from build123d import *

# Parameters (mm, degrees)
EXTRUDE_1_DEPTH              = 5
FILLET_1_R                   = 9
FILLET_2_R                   = 18
SHELL_1_T                    = -2
SKETCH_2_W                   = 27
SKETCH_2_H                   = 27
EXTRUDE_2_DEPTH              = 1
SKETCH_3_R                   = 3.975
EXTRUDE_3_DEPTH              = 1
FILLET_3_R                   = 3
HOLE_WIZARD_M2_1_D           = 2.1
HOLE_WIZARD_M2_1_CBORE_D     = 3.8
HOLE_WIZARD_M2_1_CBORE_DEPTH = 1
PATTERN_CIRCULAR_1_COUNT     = 4
SKETCH_6_R                   = 3.975
CUT_EXTRUDE_1_DEPTH          = 1
SKETCH_7_R                   = 2.5
CUT_EXTRUDE_2_DEPTH          = 2


with BuildPart() as part:
    # ｽｹｯﾁ1 → ﾎﾞｽ - 押し出し1 (new body)
    with BuildSketch(Plane(origin=(0, 0, 0), x_dir=(1, 0, 0), z_dir=(0, 1, 0))):
        with BuildLine():
            Line((-20, 50), (28.833147735, 50))
            ThreePointArc((28.833147735, 50), (44, 0), (28.833147735, -50))
            Line((28.833147735, -50), (-20, -50))
            Line((-20, -50), (-20, 50))
        make_face()
    extrude(amount=EXTRUDE_1_DEPTH)

    # ﾌｨﾚｯﾄ1
    fillet_1_edges = [part.edges().sort_by_distance(p)[0] for p in [
        (-20, 2.5, -50),
        (-20, 2.5, 50),
    ]]
    fillet(fillet_1_edges, radius=FILLET_1_R)

    # ﾌｨﾚｯﾄ2
    fillet_2_edges = [part.edges().sort_by_distance(p)[0] for p in [
        (28.833147735, 2.5, -50),
        (28.833147735, 2.5, 50),
    ]]
    fillet(fillet_2_edges, radius=FILLET_2_R)

    # ｼｪﾙ1
    shell_1_openings = [part.faces().sort_by_distance(p)[0] for p in [
        (9.782139289, 5, 0),
    ]]
    offset(amount=SHELL_1_T, openings=shell_1_openings, kind=Kind.INTERSECTION)

    # ｽｹｯﾁ2 → ﾎﾞｽ - 押し出し2 (add)
    with BuildSketch(Plane(origin=(0, 2, 0), x_dir=(1, 0, 0), z_dir=(0, 1, 0))):
        Rectangle(SKETCH_2_W, SKETCH_2_H)
    extrude(amount=EXTRUDE_2_DEPTH)

    # ｽｹｯﾁ3 → ﾎﾞｽ - 押し出し3 (add)
    with BuildSketch(Plane(origin=(0, 3, 0), x_dir=(1, 0, 0), z_dir=(0, 1, 0))):
        with Locations(Location((0, 0, 0), (0, 0, 270))):
            Circle(SKETCH_3_R)
    extrude(amount=EXTRUDE_3_DEPTH)

    # ﾌｨﾚｯﾄ3
    fillet_3_edges = [part.edges().sort_by_distance(p)[0] for p in [
        (13.5, 2.5, 13.5),
        (13.5, 2.5, -13.5),
        (-13.5, 2.5, -13.5),
        (-13.5, 2.5, 13.5),
    ]]
    fillet(fillet_3_edges, radius=FILLET_3_R)

    # M2 なべ頭ねじ用座ぐり穴1 (through all)
    with Locations(Plane(origin=(0, 0, 0), x_dir=(-1, 0, 0), z_dir=(0, -1, 0))):
        with Locations((10.5, 10.5)):
            hole_wizard_m2_1 = CounterBoreHole(HOLE_WIZARD_M2_1_D / 2, HOLE_WIZARD_M2_1_CBORE_D / 2, HOLE_WIZARD_M2_1_CBORE_DEPTH)

    # 円形ﾊﾟﾀｰﾝ1: M2 なべ頭ねじ用座ぐり穴1 ×4 about axis
    pattern_circular_1_axis = Axis((0, 0, 0), (0, 1, 0))
    for i in range(1, PATTERN_CIRCULAR_1_COUNT):
        add(hole_wizard_m2_1.rotate(pattern_circular_1_axis, i * 360 / PATTERN_CIRCULAR_1_COUNT), mode=Mode.SUBTRACT)

    # ｽｹｯﾁ6 → ｶｯﾄ - 押し出し1 (cut)
    with BuildSketch(Plane(origin=(0, 3, 0), x_dir=(1, 0, 0), z_dir=(0, 1, 0))):
        with BuildLine():
            Line((-7.994506037, -12.15), (7.994506037, -12.15))
            ThreePointArc((7.994506037, -12.15), (8.378679656, -8.378679656), (12.15, -7.994506037))
            Line((12.15, -7.994506037), (12.15, 7.994506037))
            ThreePointArc((12.15, 7.994506037), (8.378679656, 8.378679656), (7.994506037, 12.15))
            Line((7.994506037, 12.15), (-7.994506037, 12.15))
            ThreePointArc((-7.994506037, 12.15), (-7.62628447, 11.36125435), (-7.5, 10.5))
            ThreePointArc((-7.5, 10.5), (-9.076975053, 7.858977471), (-12.15, 7.994506037))
            Line((-12.15, 7.994506037), (-12.15, -7.994506037))
            ThreePointArc((-12.15, -7.994506037), (-9.076975053, -7.858977471), (-7.5, -10.5))
            ThreePointArc((-7.5, -10.5), (-7.62628447, -11.36125435), (-7.994506037, -12.15))
        make_face()
        with Locations(Location((0, 0, 0), (0, 0, 270))):
            Circle(SKETCH_6_R, mode=Mode.SUBTRACT)
    extrude(amount=-CUT_EXTRUDE_1_DEPTH, mode=Mode.SUBTRACT)

    # ｽｹｯﾁ7 → ｶｯﾄ - 押し出し2 (cut)
    with BuildSketch(Plane(origin=(0, 4, 0), x_dir=(1, 0, 0), z_dir=(0, 1, 0))):
        with Locations(Location((0, 0, 0), (0, 0, 270))):
            Circle(SKETCH_7_R)
    extrude(amount=-CUT_EXTRUDE_2_DEPTH, mode=Mode.SUBTRACT)


solid = part.part
Could you check a few things on this model? Use its own coordinates, in mm. A direction names the side the tool comes from. Coordinates: 2 decimals unless noted, no trailing zeros. Loops run counter-clockwise (first coordinate to the right, second up) from the corner with the lowest first, then second, coordinate; pieces in that order, holes last. Notation, with made-up numbers: (29.25, 45.25) -> (45.25, 45.25) arc R11 ccw to (45.25, 66.25) -> close; hole circle Ø4 at (74.5, 20). An arc over 180 degrees is marked (long way). Answer in a Markdown table with one row per item.
(1) Imagine slicing it at B-B (x = 19.5). List the corners of the cut face in (y, z) for me, plus the area to 3 significant figures.
Results found:
| item | result |
|---|---|
| outline | (0, -49.97) -> (5, -49.97) -> (5, -47.97) -> (2, -47.97) -> (2, 47.97) -> (5, 47.97) -> (5, 49.97) -> (0, 49.97) -> close |
| area | 212 mm^2 |
(2) If I drill on probe 1 along Z at (x, y) = (-10.5, 2.1); probe 2 along Z at (x, y) = (-10.5, 1.5); probe 3 along X at (y, z) = (1.6, -10.5), over which ranges is the centre line in solid material (lowest first)?
Results found:
| item | result |
|---|---|
| probe 1 | z = -50 to -48, -13.5 to -11.55, -9.45 to -7.5, 7.5 to 9.45, 11.55 to 13.5, 48 to 50 |
| probe 2 | z = -50 to -11.55, -9.45 to 9.45, 11.55 to 50 |
| probe 3 | x = -20 to -11.55, -9.45 to 9.45, 11.55 to 43.39 |
(3) Thinking about a two-plate mould opening in X: for faces 4 (the face through (12, 0, -1)), 5 (the face through (12, 1, 11)), 6 (the face through (-20, 2, 1)), which applies, released by +X, released by -X, zero draft, split by the parting line, or undercut?
Results found:
| item | result |
|---|---|
| face 4 | zero draft |
| face 5 | undercut |
| face 6 | released by -X |
(4) Will these pins go through, and if not, where does the flat tip stop? pin 1 Ø1.5 at (x, z) = (-3, -2.5) entering from +Y; pin 2 Ø1 at (x, y) = (22.5, 3) entering from -Z; pin 3 Ø2.5 at (x, z) = (-10.5, -10.5) entering from +Y; pin 4 Ø1.3 at (x, z) = (10.5, 10.5) entering from +Y.
Results found:
| item | result |
|---|---|
| pin 1 | stops at y = 4 |
| pin 2 | stops at z = -49.66 |
| pin 3 | stops at y = 3 |
| pin 4 | passes through |
(5) Imagine slicing it at A-A (z = 0). List the corners of the cut face in (x, y) for me (3 decimals).
Results found:
| item | result |
|---|---|
| outline | (-20, 0) -> (44, 0) -> (44, 5) -> (42, 5) -> (42, 2) -> (13.5, 2) -> (13.5, 3) -> (12.15, 3) -> (12.15, 2) -> (3.975, 2) -> (3.975, 4) -> (2.5, 4) -> (2.5, 2) -> (-2.5, 2) -> (-2.5, 4) -> (-3.975, 4) -> (-3.975, 2) -> (-12.15, 2) -> (-12.15, 3) -> (-13.5, 3) -> (-13.5, 2) -> (-18, 2) -> (-18, 5) -> (-20, 5) -> close |
(6) For faces 1 (the face through (28.103, 2.535, 47.223)), 2 (the face through (-12, 1, -11)), 3 (the face through (42, 3.48, -0.57)), which set-ups out of +Z, -Z, +X, -X, +Y, -Y let a thin tool reach every point of the face, with its end or its side?
Results found:
| item | result |
|---|---|
| face 1 | +Z, +X, +Y, -Y |
| face 2 | -Y |
| face 3 | +Y |
